```python
from build123d import *

# Parameters (mm, degrees)
SKETCH008_R     = 1.6
SKETCH008_R_2   = 1.5
PAD002_DEPTH    = 28
SKETCH018_W     = 29
SKETCH018_H     = 20
POCKET011_DEPTH = 42
SKETCH020_W     = 23
SKETCH020_H     = 20
POCKET013_DEPTH = 31
SKETCH021_W     = 28
SKETCH021_H     = 20
POCKET014_DEPTH = 11
SKETCH022_R     = 3.2
POCKET015_DEPTH = 5
SKETCH023_R     = 4
SKETCH023_R_2   = 1.6
POCKET016_DEPTH = 5


with BuildPart() as part:
    # Sketch008 → Pad002 (new body)
    with BuildSketch(Plane.XY):
        Polygon((-14, -17), (-10, -21), (42, -21), (44, -19), (44, -5), (42, -3), (23, -3), (3, 10), (-11, 10), (-14, 7), align=None)
        with Locations((28, -11)):
            Circle(SKETCH008_R, mode=Mode.SUBTRACT)
        with Locations((39, -11)):
            Circle(SKETCH008_R_2, mode=Mode.SUBTRACT)
    extrude(amount=PAD002_DEPTH)

    # Sketch018 (on Face6 of Pad002) → Pocket011 (cut)
    with BuildSketch(Plane.XZ.offset(21)):
        with Locations((35.5, 14)):
            Rectangle(SKETCH018_W, SKETCH018_H)
    extrude(amount=-POCKET011_DEPTH, mode=Mode.SUBTRACT)

    # Sketch020 → Pocket013 (cut)
    with BuildSketch(Plane.YZ.offset(21)):
        with Locations((5.5, 14)):
            Rectangle(SKETCH020_W, SKETCH020_H)
    extrude(amount=-POCKET013_DEPTH, mode=Mode.SUBTRACT)

    # Sketch021 (on Face17 of Pocket013) → Pocket014 (cut)
    with BuildSketch(Plane(origin=(0, -6, 0), x_dir=(-1, 0, 0), z_dir=(0, 1, 0))):
        with Locations((-4, 14)):
            Rectangle(SKETCH021_W, SKETCH021_H)
    extrude(amount=-POCKET014_DEPTH, mode=Mode.SUBTRACT)

    # Sketch022 (on Face16 of Pocket014) → Pocket015 (cut)
    with BuildSketch(Plane.YZ.offset(21)):
        with Locations((-11, 14)):
            Circle(SKETCH022_R)
    extrude(amount=-POCKET015_DEPTH, mode=Mode.SUBTRACT)

    # Sketch023 (on Face7 of Pocket015) → Pocket016 (cut)
    with BuildSketch(Plane(origin=(-14, 0, 0), x_dir=(0, -1, 0), z_dir=(-1, 0, 0))):
        with Locations((11, 14)):
            Circle(SKETCH023_R)
        with Locations((-0.5, 14)):
            Circle(SKETCH023_R_2)
    extrude(amount=-POCKET016_DEPTH, mode=Mode.SUBTRACT)


solid = part.part
```
Input: part model. Units: mm. Frame: model coordinates. A direction names the side the tool comes from. Round coordinates to 2 decimals unless told otherwise and drop trailing zeros. Loops run counter-clockwise (first coordinate to the right, second up) from the corner with the lowest first, then second, coordinate; pieces in that order, holes last. Notation, with made-up numbers: (54.5, -19) -> (110.5, -19) arc R26 cw to (110.5, 2) -> close; hole circle Ø8 at (6, 4.25). An arc over 180 degrees is marked (long way). One line per item, written item: value.
(1) Set-up query: faces 4 (the face through (4, -17, 14)), 5 (the face through (33, -3, 2)), 6 (the face through (44, -12, 2)). Return all of +Z, -Z, +X, -X, +Y, -Y with unobstructed straight access to the full face (end or side cutting, diameter ignored); none if empty.
Geometry check:
face 4: +Y
face 5: +Z, -Z, +X, +Y
face 6: +Z, -Z, +X, +Y, -Y
(2) Pin query (flat end, axial travel): pin 1 (1.5 mm diameter, centred on x = 5.5, z = 23, fed in from +Y); pin 2 (3 mm diameter, centred on x = 29, z = 2, fed in from +Y); pin 3 (2.5 mm diameter, centred on x = 19.5, z = 16.5, fed in from +Y). Return the tip coordinate at first contact, or that it passes through.
Geometry check:
pin 1: y = -17
pin 2: y = -3
pin 3: y = -6
(3) Section A-A (x = 39). Return the cut outline in (y, z).
Geometry check:
outline: (-21, 0) -> (-12.5, 0) -> (-12.5, 4) -> (-21, 4) -> close; (-21, 24) -> (-12.5, 24) -> (-12.5, 28) -> (-21, 28) -> close; (-9.5, 0) -> (-3, 0) -> (-3, 4) -> (-9.5, 4) -> close; (-9.5, 24) -> (-3, 24) -> (-3, 28) -> (-9.5, 28) -> close
(4) Material intervals for line 1 (Z direction, x = -3, y = 6); line 2 (X direction, y = -11, z = 26.95); line 3 (Z direction, x = 19.3, y = -11), sorted ascending. Write a range as [from, to].
Geometry check:
line 1: [0, 4], [24, 28]
line 2: [-14, 26.4], [29.6, 37.5], [40.5, 44]
line 3: [0, 10.8], [17.2, 28]
(5) Section D-D (y = -18). Return the cut outline in (x, z), plus the area to 3 significant figures.
Geometry check:
outline: (-13, 0) -> (44, 0) -> (44, 4) -> (21, 4) -> (21, 24) -> (44, 24) -> (44, 28) -> (-13, 28) -> close
area: 1,140 mm2
(6) Mould query, pull axis Y, two halves, no side actions, for faces 1 (the face through (21, -15, 14)), 2 (the face through (37.8, -11.9, 2)), 3 (the face through (-10.2, 10, 13.9)). Classes: pulls with the +Y half, pulls with the -Y half, needs draft (parallel to the pull), parting line crosses it, or undercut.
Geometry check:
face 1: needs draft
face 2: undercut
face 3: pulls with the +Y half
(7) Section C-C (x = 19). Return the cut outline in (y, z).
Geometry check:
outline: (-21, 0) -> (-0.4, 0) -> (-0.4, 4) -> (-6, 4) -> (-6, 24) -> (-0.4, 24) -> (-0.4, 28) -> (-21, 28) -> close; hole circle Ø6.4 at (-11, 14)
(8) Section B-B (z = 14). Return the cut outline in (x, y).
Geometry check:
outline: (-14, -17) -> (-10, -21) -> (21, -21) -> (21, -14.2) -> (18, -14.2) -> (18, -17) -> (-10, -17) -> (-10, -15) -> (-14, -15) -> close; (-14, -7) -> (-10, -7) -> (-10, -1.1) -> (-14, -1.1) -> close; (-14, 2.1) -> (-10, 2.1) -> (-10, 10) -> (-11, 10) -> (-14, 7) -> close; (18, -7.8) -> (21, -7.8) -> (21, -6) -> (18, -6) -> close
